Here's how the part is built. I have some questions about the finished solid (model axes, mm). Coordinates: 2 decimals unless noted, no trailing zeros. Order: outer loops, then holes, each group sorted by start corner. A loop starts at its lowest first (then second) coordinate and runs counter-clockwise, first axis right, second up. Notation, with made-up numbers: (8.25, -20.75) - (63.25, -20.75) arc R19 ccw to (63.25, 13.25) - close; hole circle Ø6 at (-3.75, -20). An arc over 180 degrees is marked (long way). Use one line per item in the form item = value. Start each with the question number.
Autodesk Inventor part; units mm, degrees
ref_plane "YZ Plane" through (0, 0, 0) normal (1, 0, 0) x (0, 1, 0)
ref_plane "XZ Plane" through (0, 0, 0) normal (0, 1, 0) x (-1, 0, 0)
ref_plane "XY Plane" through (0, 0, 0) normal (0, 0, 1) x (1, 0, 0)
sketch "Sketch1" plane through (0, 0, 0) normal (0, 0, 1) x (1, 0, 0)
  line L0 (-50, 26) -> (50, 26)
  line L1 (50, 26) -> (50, -26)
  line L2 (50, -26) -> (-50, -26)
  line L3 (-50, -26) -> (-50, 26)
  point P0 (0, 0)
  dimension "d0" = 100
  dimension "d1" = 52
  dimension "d2" = 50
  dimension "d3" = 26
extrude "Extrusion1" add sketch "Sketch1" along normal blind 1.6
sketch "Sketch2" plane through (0, 0, 1.6) normal (0, 0, 1) x (1, 0, 0)
  line L0 (-50, 26) -> (-50, -26)
  line L1 (-50, -26) -> (50, -26)
  point P0 (0, 0)
  point P1 (-47, -23)
  point P2 (0, -23)
  point P3 (-47, 23)
  point P4 (47, 23)
  point P5 (47, -11)
  dimension "d6" = 3
  dimension "d7" = 3
  dimension "d8" = 50
  dimension "d9" = 3
  dimension "d10" = 97
  dimension "d11" = 15
  dimension "d12" = 3
  dimension "d13" = 49
  dimension "d14" = 97
  dimension "d15" = 49
hole "Hole1" at (-47, -23, 1.6) at (0, -23, 1.6) at (-47, 23, 1.6) at (47, 23, 1.6) at (47, -11, 1.6) direction (0, 0, -1) diameter 2.1 depth 10 tip angle 118
sketch "Sketch3" plane through (0, 0, 1.6) normal (0, 0, 1) x (1, 0, 0)
  line L0 (-50, -26) -> (50, -26)
  line L1 (-42.3, -26) -> (-3.6, -26)
  line L2 (-3.6, -26) -> (-3.6, -19.3)
  line L3 (-3.6, -19.3) -> (-42.3, -19.3)
  line L4 (-42.3, -19.3) -> (-42.3, -26)
  line L5 (50, -26) -> (50, 26)
  line L6 (13.1, -26) -> (50, -26)
  line L7 (50, -26) -> (50, -13.5)
  line L8 (50, -13.5) -> (13.1, -13.5)
  line L9 (13.1, -13.5) -> (13.1, -26)
  line L10 (13.1, -13.5) -> (0.7, -26)
  line L11 (0.7, -26) -> (13.1, -26)
  line L12 (-50, 26) -> (-50, -26)
  point P0 (0, 0)
  dimension "d23" = 7.7
  dimension "d24" = 6.7
  dimension "d25" = 46.4
  dimension "d26" = 50.7
  dimension "d27" = 63.1
  dimension "d28" = 12.5
extrude "Extrusion2" cut sketch "Sketch3" against normal blind 1.6
fillet "Fillet1" radius 3 4 edges at (-50, -26, 0.8) (-50, 26, 0.8) (50, -13.5, 0.8) (50, 26, 0.8)
properties part number "pcb_mockup"
1) Suppose I cut it at B-B, the plane x = 31. List the corners of the cut face in (y, z) for me, then the cut area to 3 significant figures.
2) For pin 1 (0.8 mm diameter, centred on y = -24, z = 1, fed in from +X); pin 2 (0.5 mm diameter, centred on x = 21.5, z = 1, fed in from -Y); pin 3 (6 mm diameter, centred on x = -35.5, y = -4.5, fed in from -Z), each with a flat end and sliding along its axis, tell me the tip position at first contact or that it passes through.
3) I need wall thicknesses on probe 1 along X at (y, z) = (23, 0.9); probe 2 along Y at (x, z) = (-47, 0.6); probe 3 along Y at (x, z) = (0, 0.9). Which ranges of each line are inside material? Lowest first, please. Write a range as [from, to].
4) If we mould it in two halves opening along X, with no side actions, what happens to faces 1 (the flat face through (6.99, -19.66, 0.81)), 2 (the flat face through (-1, 6, 0)), 3 (the cylindrical face through (-46.6, -23.97, 0.79))? For each: pulls with the +X half, pulls with the -X half, needs draft (parallel to the pull), parting line crosses it, or undercut.
5) Suppose I cut it at A-A, the plane z = 1.35. List the corners of the cut face in (x, y) for me, then the cut area to 3 significant figures.
6) Suppose I cut it at C-C, the plane x = -21. List the corners of the cut face in (y, z) for me, then the cut area to 3 significant figures.
From the geometry:
q1.outline = (-13.5, 0) - (26, 0) - (26, 1.6) - (-13.5, 1.6) - close
q1.area = 63.2 mm2
q2.pin_1 = 3.08
q2.pin_2 = -13.5
q2.pin_3 = 0
q3.probe_1 = [-50, -48.05], [-45.95, 45.95], [48.05, 50]
q3.probe_2 = [-26, -24.05], [-21.95, 21.95], [24.05, 26]
q3.probe_3 = [-26, -24.05], [-21.95, 26]
q4.face_1 = pulls with the +X half
q4.face_2 = needs draft
q4.face_3 = undercut
q5.outline = (-50, -23) arc R3 ccw to (-47, -26) - (-42.3, -26) - (-42.3, -19.3) - (-3.6, -19.3) - (-3.6, -26) - (0.7, -26) - (13.1, -13.5) - (47, -13.5) arc R3 ccw to (50, -10.5) - (50, 23) arc R3 ccw to (47, 26) - (-47, 26) arc R3 ccw to (-50, 23) - close; hole circle Ø2.1 at (-47, -23); hole circle Ø2.1 at (-47, 23); hole circle Ø2.1 at (0, -23); hole circle Ø2.1 at (47, -11); hole circle Ø2.1 at (47, 23)
q5.area = 4,380 mm2
q6.outline = (-19.3, 0) - (26, 0) - (26, 1.6) - (-19.3, 1.6) - close
q6.area = 72.5 mm2
